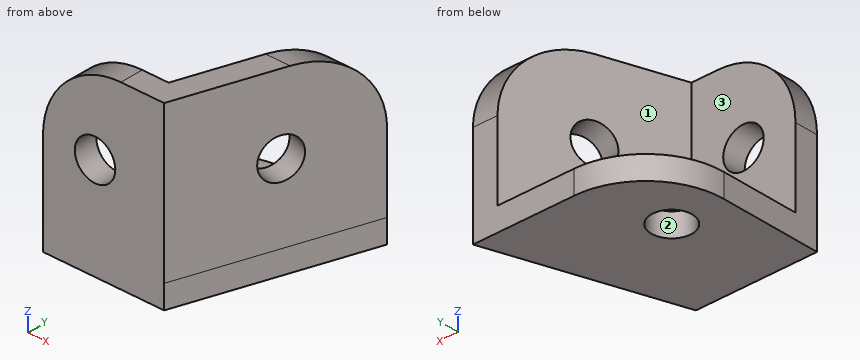
```python
from build123d import *

# Parameters (mm, degrees)
BOSS_EXTRU_1_DEPTH      = 3
ESQUISSE2_W             = 20
ESQUISSE2_H             = 24.175680092
BOSS_EXTRU_2_DEPTH      = 3
ESQUISSE3_W             = 15.552617377
ESQUISSE3_H             = 3
BOSS_EXTRU_3_DEPTH      = 20
ENL_V_MAT_EXTRU_1_DEPTH = 20
CONG_1_R                = 10
ESQUISSE5_R             = 2.6
ENL_V_MAT_EXTRU_2_DEPTH = 20
ESQUISSE6_R             = 2.6
ENL_V_MAT_EXTRU_3_DEPTH = 20
ESQUISSE7_R             = 2.6
ENL_V_MAT_EXTRU_4_DEPTH = 20


with BuildPart() as part:
    # Esquisse1 → Boss.-Extru.1 (new body)
    with BuildSketch(Plane.XY):
        Polygon((55.418780356, 3), (55.418780356, 26), (78.418780356, 26), (70.971397733, 3), align=None)
    extrude(amount=BOSS_EXTRU_1_DEPTH)

    # Esquisse2 → Boss.-Extru.2 (add)
    with BuildSketch(Plane(origin=(63.357248994, -20.515029356, 0), x_dir=(0, 0, 1), z_dir=(-0.9513693063481515, 0.30805266260598535, 0))):
        with Locations((13, 36.804876006)):
            Rectangle(ESQUISSE2_W, ESQUISSE2_H)
    extrude(amount=BOSS_EXTRU_2_DEPTH)

    # Esquisse3 → Boss.-Extru.3 (add)
    with BuildSketch(Plane.XY.offset(3)):
        with Locations((63.195089045, 4.5)):
            Rectangle(ESQUISSE3_W, ESQUISSE3_H)
    extrude(amount=BOSS_EXTRU_3_DEPTH)

    # Esquisse4 → Enlèv. mat.-Extru.1 (cut)
    with BuildSketch(Plane.XY.offset(23)):
        Polygon((78.418780356, 26), (75.265430779, 26), (75.564672437, 26.924157988), align=None)
    extrude(amount=-ENL_V_MAT_EXTRU_1_DEPTH, mode=Mode.SUBTRACT)

    # Congé1
    # the kernel refuses this fillet: 10 mm, written as the material it takes off along each edge
    with BuildSketch(Plane(origin=(55.418780356, 31, 23), x_dir=(0, 0, -1), z_dir=(0, -1, 0)), Plane(origin=(55.418780356, 26, -25), x_dir=(0, -1, 0), z_dir=(0, 0, 1))) as cong_1_piece_1:
        with BuildLine():
            CenterArc((CONG_1_R, CONG_1_R), CONG_1_R, 180, 90)
            Line((0, CONG_1_R), (0, 0))
            Line((0, 0), (CONG_1_R, 0))
        make_face()
    extrude(amount=53, mode=Mode.SUBTRACT)
    with BuildSketch(Plane(origin=(103.418780356, 26, 23), x_dir=(0, 0, -1), z_dir=(-1, 0, 0))) as cong_1_piece_2:
        with BuildLine():
            CenterArc((CONG_1_R, CONG_1_R), CONG_1_R, 180, 90)
            Line((0, CONG_1_R), (0, 0))
            Line((0, 0), (CONG_1_R, 0))
        make_face()
    extrude(amount=53.153349577, mode=Mode.SUBTRACT)

    # Esquisse5 → Enlèv. mat.-Extru.2 (cut)
    with BuildSketch(Plane.XY.offset(3)):
        with Locations((62.104113123, 16)):
            Circle(ESQUISSE5_R)
    extrude(amount=-ENL_V_MAT_EXTRU_2_DEPTH, mode=Mode.SUBTRACT)

    # Esquisse6 → Enlèv. mat.-Extru.3 (cut)
    with BuildSketch(Plane(origin=(0, 6, 0), x_dir=(1, 0, 0), z_dir=(0, 1, 0))):
        with Locations(Location((62.104113123, -13, 0), (0, 0, 270))):
            Circle(ESQUISSE6_R)
    extrude(amount=-ENL_V_MAT_EXTRU_3_DEPTH, mode=Mode.SUBTRACT)

    # Esquisse7 → Enlèv. mat.-Extru.4 (cut)
    with BuildSketch(Plane(origin=(60.503141075, -19.590871368, 0), x_dir=(0, 0, 1), z_dir=(-0.9513693063481516, 0.30805266260598513, 0))):
        with Locations(Location((13, 37.410153061, 0), (0, 0, 270))):
            Circle(ESQUISSE7_R)
    extrude(amount=-ENL_V_MAT_EXTRU_4_DEPTH, mode=Mode.SUBTRACT)


solid = part.part
```
Build history of the part. All positions in model axes, mm. Face numbers are marked on the shaded views. Coordinates: 2 decimals unless noted, no trailing zeros. Write each loop counter-clockwise with the first axis right and the second up, starting at its lowest first coordinate (ties: lowest second). Pieces come first, ordered by that corner, then holes.
1. Pull direction X, two halves, no side cores. Call the marked faces 1, 2 and 3: released by +X, released by -X, zero draft, split by the parting line, or undercut.
Answer block:
face 1: released by -X
face 2: undercut
face 3: zero draft
2. Band-saw the part on B-B, the plane z = 4.75. Give the cut face in (x, y), and give its area (3 significant figures).
Answer block:
outline: (55.42, 3) - (70.97, 3) - (78.42, 26) - (75.27, 26) - (68.79, 6) - (55.42, 6) - close
area: 111 mm2
3. Band-saw the part on A-A, the plane x = 62.5. Give the cut face in (y, z), and give its area (3 significant figures).
Answer block:
outline: (3, 0) - (13.43, 0) - (13.43, 3) - (6, 3) - (6, 10.43) - (3, 10.43) - close; (3, 15.57) - (6, 15.57) - (6, 22.56) - (3, 22.56) - close; (18.57, 0) - (25.56, 0) - (25.56, 3) - (18.57, 3) - close
area: 95.6 mm2
4. Band-saw the part on D-D, the plane x = 69.5. Give the cut face in (y, z), and give its area (3 significant figures).
Answer block:
outline: (3, 0) - (26, 0) - (26, 3) - (8.19, 3) - (8.19, 23) - (3, 23) - close
area: 173 mm2
5. Drill centre lines: probe 1 along Z at (x, y) = (57.5, 8); probe 2 along Y at (x, z) = (59.5, 9.5); probe 3 along X at (y, z) = (4.4, 13). Where is each one in solid material? Low to high.
Answer block:
probe 1: z = 0 to 3
probe 2: y = 3 to 6
probe 3: x = 55.42 to 59.5, 64.7 to 71.42
6. Band-saw the part on C-C, the plane y = 9.75. Give the cut face in (x, z), and give its area (3 significant figures).
Answer block:
outline: (55.42, 0) - (73.16, 0) - (73.16, 23) - (70, 23) - (70, 3) - (55.42, 3) - close
area: 116 mm2
7. Drop flat-ended pins along their axis: pin 1 (10 mm diameter, centred on y = 11, z = 19, fed in from +X); pin 2 (10 mm diameter, centred on x = 61, y = 19, fed in from +Z); pin 3 (6 mm diameter, centred on x = 62.1, z = 13, fed in from +Y). Give the stop position or say it passes through.
Answer block:
pin 1: stops at x = 75.18
pin 2: stops at z = 3
pin 3: stops at y = 6
